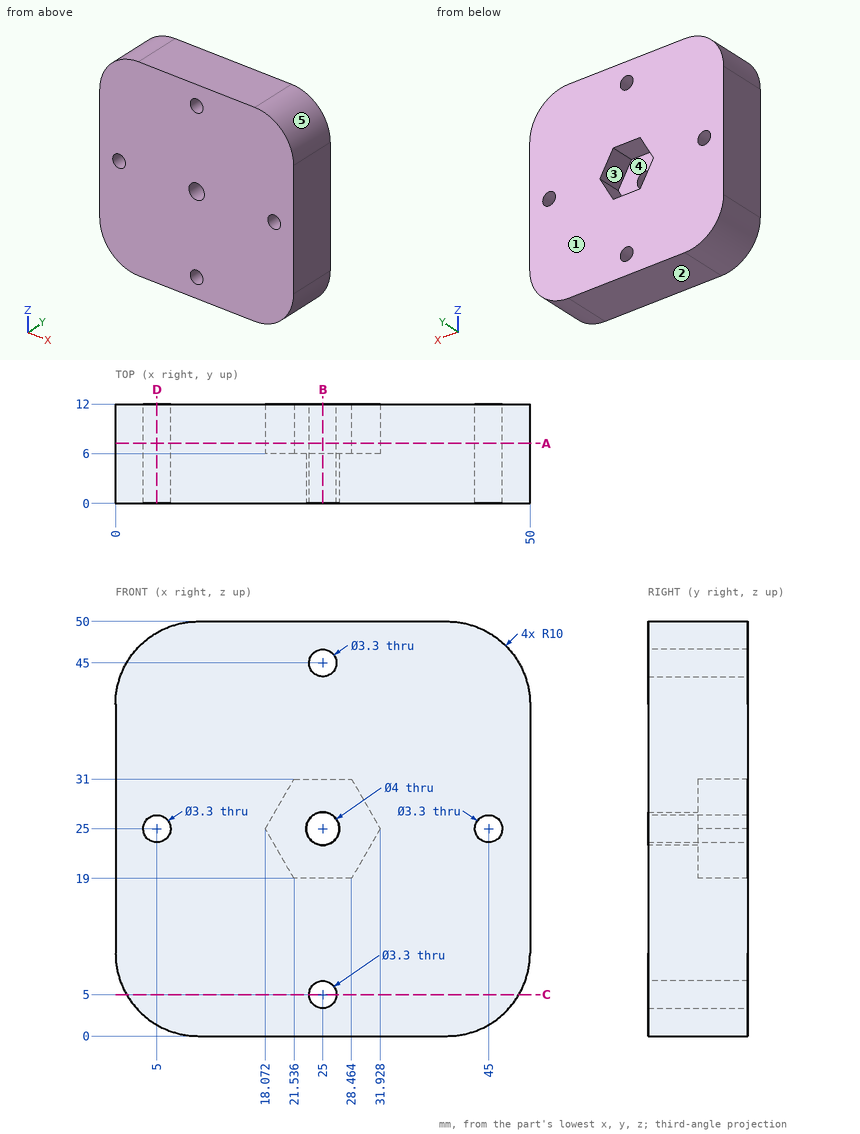
Check sheet for the drawn part. Datum: minimum x, y, z corner. Units: mm. A direction names the side the tool comes from. Give positions to 0.01 mm unless a question says otherwise; leave off trailing zeros. Order: outer loops, then holes, each group sorted by start corner. A loop starts at its lowest first (then second) coordinate and runs counter-clockwise, first axis right, second up. Notation, with made-up numbers: (39, 12.25) - (60, 12.25) arc R26 cw to (60, 48.25) - close; hole circle Ø3 at (-32, 80.25). An arc over 180 degrees is marked (long way). Answer in a Markdown table with one row per item. Add a question column.
Q1. Material ranges on probe 1 along X at (y, z) = (3.15, 25); probe 2 along X at (y, z) = (6.5, 25); probe 3 along X at (y, z) = (3, 9.5), recorded low to high. Write a range as from..to.
Q2. Cross-section at A-A, the plane y = 7.25. Enter the section's corners in (x, z), then the cut area to 3 significant figures.
Q3. Gauge pin test, flat ends, axial feed: pin 1 (1.5 mm diameter, centred on x = 21, y = 8.5, fed in from -Z); pin 2 (5 mm diameter, centred on x = 25, z = 25, fed in from +Y); pin 3 (2.5 mm diameter, centred on x = 5, z = 25, fed in from +Y). Record the tip position at first contact, or that the pin passes through.
Q4. Mould release check, pull along Z, two halves, no side actions. Record for the marked faces 1, 2 and 3: pulls with the +Z half, pulls with the -Z half, needs draft (parallel to the pull), parting line crosses it, or undercut.
Q5. Cross-section at C-C, the plane z = 5. Enter the section's corners in (x, y).
Q6. Cross-section at D-D, the plane x = 5. Enter the section's corners in (y, z).
Q7. Tool access check on the marked faces 4 and 5. Record the directions out of +Z, -Z, +X, -X, +Y, -Y that give a thin tool (end or side, any length) a straight path to the whole face; none if there is none.
Q8. Cross-section at B-B, the plane x = 25. Enter the section's corners in (y, z).
Check values:
| question | item | result |
|---|---|---|
| 1 | probe 1 | x = 0..3.35, 6.65..23, 27..43.35, 46.65..50 |
| 1 | probe 2 | x = 0..3.35, 6.65..18.07, 31.93..43.35, 46.65..50 |
| 1 | probe 3 | x = 0.01..49.99 |
| 2 | outline | (0, 10) arc R10 ccw to (10, 0) - (40, 0) arc R10 ccw to (50, 10) - (50, 40) arc R10 ccw to (40, 50) - (10, 50) arc R10 ccw to (0, 40) - close; hole circle Ø3.3 at (5, 25); hole (18.07, 25) - (21.54, 19) - (28.46, 19) - (31.93, 25) - (28.46, 31) - (21.54, 31) - close; hole circle Ø3.3 at (25, 5); hole circle Ø3.3 at (25, 45); hole circle Ø3.3 at (45, 25) |
| 2 | area | 2,260 mm^2 |
| 3 | pin 1 | stops at z = 0 |
| 3 | pin 2 | stops at y = 6 |
| 3 | pin 3 | passes through |
| 4 | face 1 | needs draft |
| 4 | face 2 | pulls with the -Z half |
| 4 | face 3 | undercut |
| 5 | outline | (1.34, 0) - (23.35, 0) - (23.35, 12) - (1.34, 12) - close; (26.65, 0) - (48.66, 0) - (48.66, 12) - (26.65, 12) - close |
| 6 | outline | (0, 1.34) - (12, 1.34) - (12, 23.35) - (0, 23.35) - close; (0, 26.65) - (12, 26.65) - (12, 48.66) - (0, 48.66) - close |
| 7 | face 4 | +Y |
| 7 | face 5 | +Z, +X, +Y, -Y |
| 8 | outline | (0, 0) - (12, 0) - (12, 3.35) - (0, 3.35) - close; (0, 6.65) - (12, 6.65) - (12, 19) - (6, 19) - (6, 23) - (0, 23) - close; (0, 27) - (6, 27) - (6, 31) - (12, 31) - (12, 43.35) - (0, 43.35) - close; (0, 46.65) - (12, 46.65) - (12, 50) - (0, 50) - close |
